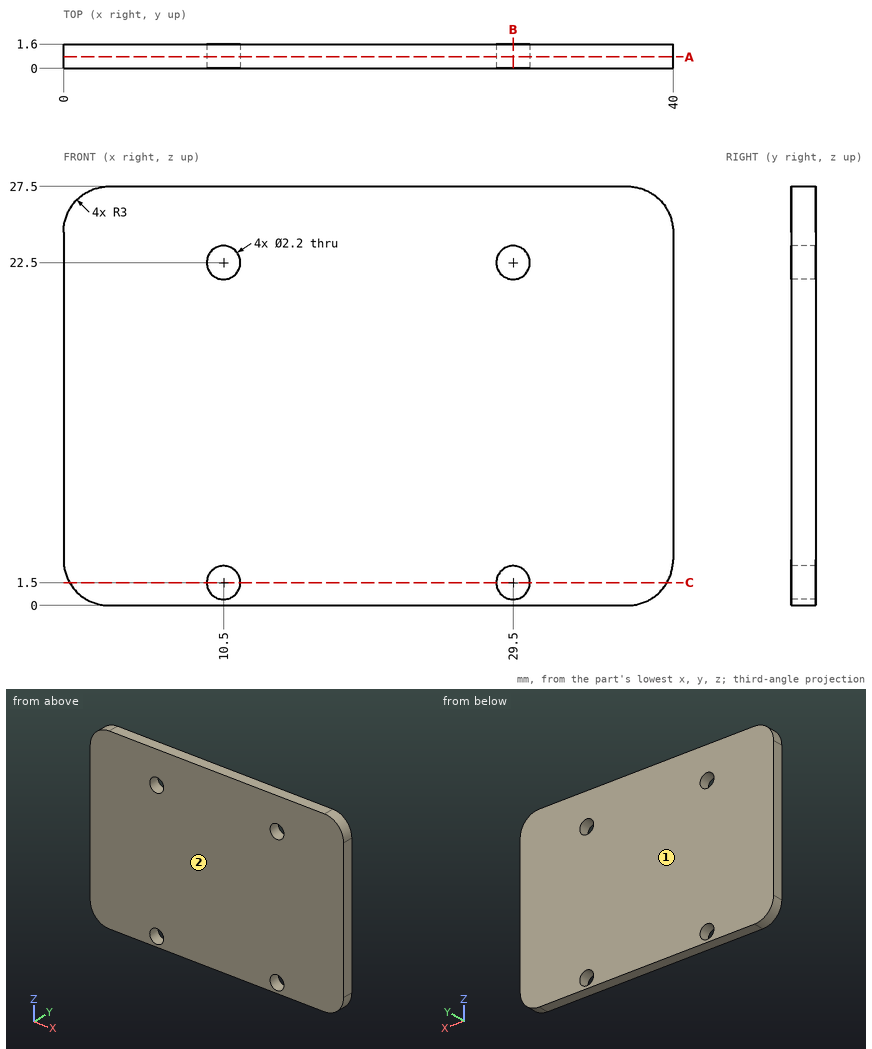
Here's the drawing with two shaded views (mm, measured from the low corner). I have some questions. Give positions to 0.01 mm unless a question says otherwise; leave off trailing zeros. Loops run counter-clockwise (first coordinate to the right, second up) from the corner with the lowest first, then second, coordinate; pieces in that order, holes last. Notation, with made-up numbers: (30.25, 43) - (45.25, 43) arc R25 ccw to (45.25, 60) - close; hole circle Ø11 at (66, -8). An arc over 180 degrees is marked (long way). Answer in a Markdown table with one row per item. Add a question column.
Q1. Please list where these lines run through material, in increasing order: L1, parallel to Z at x = 10.5, y = 1.05; L2, parallel to X at y = 0.75, z = 22.5; L3, parallel to X at y = 1.05, z = 23.25. Write a range as from..to.
Q2. We'd pull the mould along Y, two halves only. Please class the marked faces 1 and 2: +Y half, -Y half, draft (parallel to the pull), parting line (faces both ways), or undercut.
Q3. If we section it at C-C (z = 1.5): List the corners of the cut face in (x, y) for me, plus the area to 3 significant figures.
Q4. For pin 1 (1.3 mm diameter, centred on x = 10.5, z = 1.5, fed in from +Y); pin 2 (1.5 mm diameter, centred on x = 24, z = 10, fed in from -Y), each with a flat end and sliding along its axis, tell me the tip position at first contact or that it passes through.
Q5. If we section it at A-A (y = 0.75): List the corners of the cut face in (x, z) for me, plus the area to 3 significant figures.
Q6. If we section it at B-B (x = 29.5): List the corners of the cut face in (y, z) for me.
The answers:
| question | item | result |
|---|---|---|
| 1 | L1 | z = 0..0.4, 2.6..21.4, 23.6..27.5 |
| 1 | L2 | x = 0..9.4, 11.6..28.4, 30.6..40 |
| 1 | L3 | x = 0..9.7, 11.3..28.7, 30.3..40 |
| 2 | face 1 | +Y half |
| 2 | face 2 | -Y half |
| 3 | outline | (0.4, 0) - (9.4, 0) - (9.4, 1.6) - (0.4, 1.6) - close; (11.6, 0) - (28.4, 0) - (28.4, 1.6) - (11.6, 1.6) - close; (30.6, 0) - (39.6, 0) - (39.6, 1.6) - (30.6, 1.6) - close |
| 3 | area | 55.7 mm^2 |
| 4 | pin 1 | passes through |
| 4 | pin 2 | stops at y = 0 |
| 5 | outline | (0, 3) arc R3 ccw to (3, 0) - (37, 0) arc R3 ccw to (40, 3) - (40, 24.5) arc R3 ccw to (37, 27.5) - (3, 27.5) arc R3 ccw to (0, 24.5) - close; hole circle Ø2.2 at (10.5, 1.5); hole circle Ø2.2 at (10.5, 22.5); hole circle Ø2.2 at (29.5, 1.5); hole circle Ø2.2 at (29.5, 22.5) |
| 5 | area | 1,080 mm^2 |
| 6 | outline | (0, 0) - (1.6, 0) - (1.6, 0.4) - (0, 0.4) - close; (0, 2.6) - (1.6, 2.6) - (1.6, 21.4) - (0, 21.4) - close; (0, 23.6) - (1.6, 23.6) - (1.6, 27.5) - (0, 27.5) - close |
